from build123d import *

# Parameters (mm, degrees)
SKETCH1_R           = 1.6
SKETCH1_W           = 15
SKETCH1_H           = 73
SKETCH1_W_2         = 40
SKETCH1_H_2         = 15
BOSS_EXTRUDE1_DEPTH = 3
FILLET1_R           = 5


with BuildPart() as part:
    # Sketch1 → Boss-Extrude1 (new body)
    # profile 1 of 3: a face of its own
    with BuildSketch(Plane(origin=(0, 0, 0), x_dir=(1, 0, 0), z_dir=(0, 1, 0))):
        Polygon((0, 88), (12.5, 88), (27.5, 88), (40, 88), (40, 103), (0, 103), align=None)
        with Locations(Location((8, 95.5, 0), (0, 0, 270))):
            Circle(SKETCH1_R, mode=Mode.SUBTRACT)
        with Locations(Location((32, 95.5, 0), (0, 0, 270))):
            Circle(SKETCH1_R, mode=Mode.SUBTRACT)
    # profile 2 of 3: a face of its own
    with BuildSketch(Plane(origin=(0, 0, 0), x_dir=(1, 0, 0), z_dir=(0, 1, 0))):
        with Locations((20, 51.5)):
            Rectangle(SKETCH1_W, SKETCH1_H)
        with Locations(Location((20, 25, 0), (0, 0, 270))):
            Circle(SKETCH1_R, mode=Mode.SUBTRACT)
        with Locations(Location((20, 78, 0), (0, 0, 270))):
            Circle(SKETCH1_R, mode=Mode.SUBTRACT)
    # profile 3 of 3: a face of its own
    with BuildSketch(Plane(origin=(0, 0, 0), x_dir=(1, 0, 0), z_dir=(0, 1, 0))):
        with Locations((20, 7.5)):
            Rectangle(SKETCH1_W_2, SKETCH1_H_2)
        with Locations(Location((8, 7.5, 0), (0, 0, 270))):
            Circle(SKETCH1_R, mode=Mode.SUBTRACT)
        with Locations(Location((32, 7.5, 0), (0, 0, 270))):
            Circle(SKETCH1_R, mode=Mode.SUBTRACT)
    extrude(amount=BOSS_EXTRUDE1_DEPTH)

    # Fillet1
    fillet1_edges = [part.edges().sort_by_distance(p)[0] for p in [
        (40, 1.5, -88),
        (40, 1.5, -15),
        (40, 1.5, 0),
        (0, 1.5, 0),
        (0, 1.5, -15),
        (0, 1.5, -88),
        (0, 1.5, -103),
        (40, 1.5, -103),
    ]]
    fillet(fillet1_edges, radius=FILLET1_R)


solid = part.part
Build history of the part. All positions in model axes, mm. A direction names the side the tool comes from. Round coordinates to 2 decimals unless told otherwise and drop trailing zeros. Write each loop counter-clockwise with the first axis right and the second up, starting at its lowest first coordinate (ties: lowest second). Pieces come first, ordered by that corner, then holes. Notation, with made-up numbers: (-36, -12.5) - (-19, -12.5) arc R23 ccw to (-19, 10.5) - close; hole circle Ø3 at (-2.5, 76). An arc over 180 degrees is marked (long way). Use CSV: the item, a comma, the result in double quotes.
(1) Mould opens along X. For faces 4 (the cylindrical face through (1, 2, -101)), 5 (the cylindrical face through (21.586, 1.479, -25.208)), 6 (the flat face through (27.5, 1, -51)), 7 (the cylindrical face through (6.44, 1.48, -7.85)) say: pulls with the +X half, pulls with the -X half, needs draft (parallel to the pull), parting line crosses it, or undercut.
Response:
face 4,"pulls with the -X half"
face 5,"undercut"
face 6,"pulls with the +X half"
face 7,"undercut"
(2) Wall check: line 1 (X direction, y = 1.55, z = -95.5); line 2 (Z direction, x = 29, y = 0.35); line 3 (X direction, y = 1.6, z = -25). Give the ranges that are in metal, low to high.
Response:
line 1,"0 to 6.4, 9.6 to 30.4, 33.6 to 40"
line 2,"-103 to -88, -15 to 0"
line 3,"12.5 to 18.4, 21.6 to 27.5"
(3) Band-saw the part on B-B (x = 20). Write the cut outline in (y, z).
Response:
outline,"(0, -103) - (3, -103) - (3, -79.6) - (0, -79.6) - close; (0, -76.4) - (3, -76.4) - (3, -26.6) - (0, -26.6) - close; (0, -23.4) - (3, -23.4) - (3, 0) - (0, 0) - close"
(4) Band-saw the part on C-C (y = 1.2). Write the cut outline in (x, z).
Response:
outline,"(0, -98) arc R5 ccw to (5, -103) - (35, -103) arc R5 ccw to (40, -98) - (40, -93) arc R5 ccw to (35, -88) - (27.5, -88) - (27.5, -15) - (35, -15) arc R5 ccw to (40, -10) - (40, -5) arc R5 ccw to (35, 0) - (5, 0) arc R5 ccw to (0, -5) - (0, -10) arc R5 ccw to (5, -15) - (12.5, -15) - (12.5, -88) - (5, -88) arc R5 ccw to (0, -93) - close; hole circle Ø3.2 at (8, -95.5); hole circle Ø3.2 at (8, -7.5); hole circle Ø3.2 at (20, -78); hole circle Ø3.2 at (20, -25); hole circle Ø3.2 at (32, -95.5); hole circle Ø3.2 at (32, -7.5)"
(5) Band-saw the part on D-D (z = -78). Write the cut outline in (x, y), plus the area to 3 significant figures.
Response:
outline,"(12.5, 0) - (18.4, 0) - (18.4, 3) - (12.5, 3) - close; (21.6, 0) - (27.5, 0) - (27.5, 3) - (21.6, 3) - close"
area,"35.4 mm²"
(6) 3-axis set-ups, long thin cutter, end or side, ignore diameter. For faces 1 (the flat face through (20, 1, 0)), 2 (the flat face through (31, 1, -88)), 3 (the flat face through (9, 1, -15)): which of +Z, -Z, +X, -X, +Y, -Y reach the whole face in a straight line?
Response:
face 1,"+Z, +X, -X, +Y, -Y"
face 2,"+X, +Y, -Y"
face 3,"-X, +Y, -Y"
(7) Pin check, flat tips, straight feed: P1, Ø1.9, axis at x = 20, z = -78, coming from the +Y side; P2, Ø6, axis at x = 21, z = -24, coming from the -Y side; P3, Ø1, axis at y = 2, z = -37.5, coming from the -X side. Stop position of each tip, or through.
Response:
P1,"through"
P2,"y = 0"
P3,"x = 12.5"
(8) Band-saw the part on A-A (z = -7.5). Write the cut outline in (x, y).
Response:
outline,"(0, 0) - (6.4, 0) - (6.4, 3) - (0, 3) - close; (9.6, 0) - (30.4, 0) - (30.4, 3) - (9.6, 3) - close; (33.6, 0) - (40, 0) - (40, 3) - (33.6, 3) - close"
